Build history of the part. All positions in model axes, mm. Face numbers are marked on the shaded views. A direction names the side the tool comes from. Coordinates: 2 decimals unless noted, no trailing zeros. Loops run counter-clockwise (first coordinate to the right, second up) from the corner with the lowest first, then second, coordinate; pieces in that order, holes last.
(1) Slice it at C-C (z = 1.2). Give the cut face in (x, y), and give its area (3 significant figures).
(2) Two-plate mould, pull along X, no slides. Class the marked faces 3, 4 and 5: pulls with the +X half, pulls with the -X half, needs draft (parallel to the pull), parting line crosses it, or undercut.
(3) Flat gauge pins, fed straight in: P1, Ø1.5, axis at y = -1.5, z = 3, coming from the +X side; P2, Ø2, axis at y = 1.5, z = 3, coming from the -X side; P3, Ø1.5, axis at y = -3, z = 3.5, coming from the -X side. Where does each tip first touch, or does it go through?
(4) Wall check: L1, parallel to Y at x = 0, z = 2; L2, parallel to Y at x = 0, z = 0.5; L3, parallel to X at y = -1.5, z = 1.15. Give the ranges that are in metal, low to high.
(5) Slice it at D-D (z = 3.2). Give the cut face in (x, y).
(6) Slice it at A-A (y = 0). Give the cut face in (x, z), and give its area (3 significant figures).
(7) Tool access for the marked faces 1 and 2: list every direction of +Z, -Z, +X, -X, +Y, -Y with a clear straight run to the whole face (end or side of a thin tool).
from build123d import *


with BuildPart() as f1:
    # F0 (on Front) → F1 (revolve)
    with BuildSketch(Plane.XZ):
        with BuildLine():
            ThreePointArc((3, 0), (3.707107, 0.292893), (4, 1))
            Line((4, 1), (4, 2.5))
            ThreePointArc((4, 2.5), (3.414214, 3.914214), (2, 4.5))
            Line((2, 4.5), (0, 4.5))
            Line((0, 4.5), (0, 3))
            Line((0, 3), (1.75, 3))
            Line((1.75, 3), (1.75, 0.685272))
            Line((1.75, 0.685272), (1.951956, 0))
            Line((1.951956, 0), (3, 0))
        make_face()
    revolve(axis=Axis((0, 0, 144.955611), (0, 0, 1)))


solid = f1.part
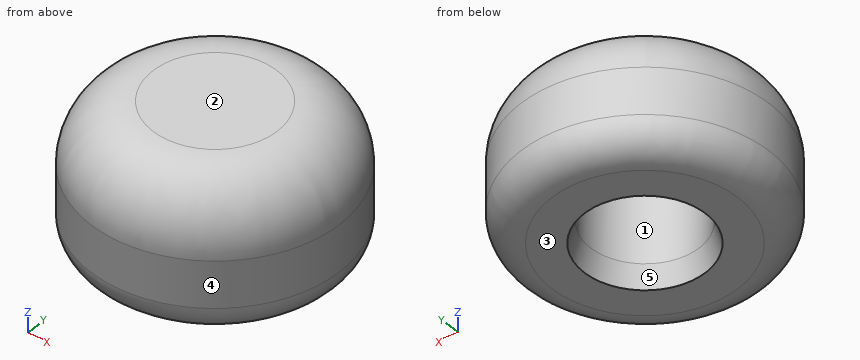
Response values:
1. outline: circle Ø8 at (0, 0); hole circle Ø3.5 at (0, 0)
1. area: 40.6 mm2
2. face 3: needs draft
2. face 4: parting line crosses it
2. face 5: undercut
3. P1: stops at x = 3.91
3. P2: stops at x = -3.95
3. P3: stops at x = -3.11
4. L1: y = -4 to -1.75, 1.75 to 4
4. L2: y = -3.87 to -1.8, 1.8 to 3.87
4. L3: x = -3.71 to -0.9, 0.9 to 3.71
5. outline: circle Ø7.75 at (0, 0)
6. outline: (-4, 1) arc R1 ccw to (-3, 0) - (-1.95, 0) - (-1.75, 0.69) - (-1.75, 3) - (1.75, 3) - (1.75, 0.69) - (1.95, 0) - (3, 0) arc R1 ccw to (4, 1) - (4, 2.5) arc R2 ccw to (2, 4.5) - (-2, 4.5) arc R2 ccw to (-4, 2.5) - close
6. area: 23.2 mm2
7. face 1: -Z
7. face 2: +Z, +X, -X, +Y, -Y
